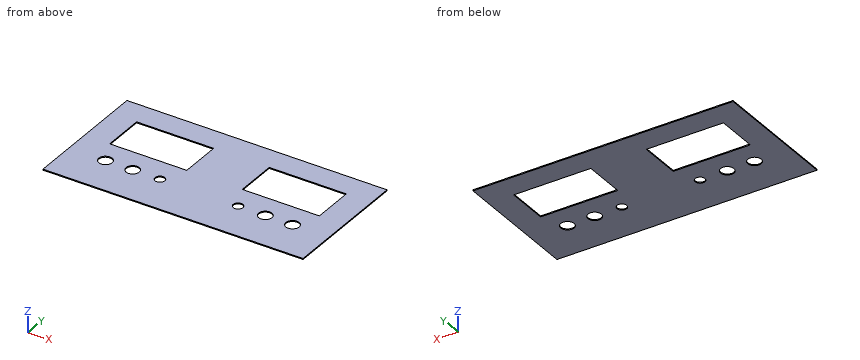
from build123d import *

# Parameters (mm, degrees)
SKETCH1_W          = 253
SKETCH1_H          = 126
BASE_FLANGE1_DEPTH = 1
SKETCH2_R          = 6.5
SKETCH2_R_2        = 4.75
SKETCH2_W          = 75
SKETCH2_H          = 40.400000001
SKETCH2_H_2        = 40.4
CUT_EXTRUDE1_DEPTH = 10


# Sheet-metal steps are written as plain solids
with BuildPart() as part:
    # Sketch1 → Base-Flange1 (new body)
    with BuildSketch(Plane.XY):
        Rectangle(SKETCH1_W, SKETCH1_H)
    extrude(amount=-BASE_FLANGE1_DEPTH)

    # Sketch2 → Cut-Extrude1 (cut)
    with BuildSketch(Plane(origin=(0, 0, -1), x_dir=(-1, 0, 0), z_dir=(0, 0, -1))):
        with Locations((-91, -24)):
            Circle(SKETCH2_R)
        with Locations((-64.5, -24)):
            Circle(SKETCH2_R)
        with Locations((64.5, -24)):
            Circle(SKETCH2_R)
        with Locations((91, -24)):
            Circle(SKETCH2_R)
        with Locations((-38, -24)):
            Circle(SKETCH2_R_2)
        with Locations((38, -24)):
            Circle(SKETCH2_R_2)
        with Locations((-64.5, 19.5)):
            Rectangle(SKETCH2_W, SKETCH2_H)
        with Locations((64.5, 19.5)):
            Rectangle(SKETCH2_W, SKETCH2_H_2)
    extrude(amount=-CUT_EXTRUDE1_DEPTH, mode=Mode.SUBTRACT)


solid = part.part
The model under review builds one solid part; all positions refer to its coordinate system, in mm. Round coordinates to 2 decimals unless told otherwise and drop trailing zeros. Loops run counter-clockwise (first coordinate to the right, second up) from the corner with the lowest first, then second, coordinate; pieces in that order, holes last. Notation, with made-up numbers: M 30.25,32.25 L 71.25,32.25 A9 ccw 71.25,42.25 Z; hole C 38,72 d3. An arc over 180 degrees is marked long. Answer as CSV lines item,"result". Start each with the question number.
Item 1: Consider section A-A (x = 77). Write out the cut boundary in (y, z).
Item 2: Wall thickness on line 1 (X direction, y = 21.5, z = -0.05); line 2 (Y direction, x = -91, z = -0.75); line 3 (Y direction, x = -92, z = -0.25): over which ranges is each line inside the solid? List them lowest first. Write a range as [from, to].
Item 3: Consider section B-B (y = -24). Write out the cut boundary in (x, z), then the cut area to 3 significant figures.
Item 4: Insertion check: P1, Ø10.5, axis at x = 91, y = -24, coming from the +Z side. The pin has a flat end and moves straight along its axis. Give the tip position at first contact, or say it passes through.
Item 5: Consider section D-D (z = -0.6). State how many separate pieces and enclosed holes the cut face has, then the cut area to 3 significant figures.
Item 6: Consider section C-C (x = -91). Write out the cut boundary in (y, z), then the cut area to 3 significant figures.
Answer:
1,outline,"M -63,-1 L -0.7,-1 L -0.7,0 L -63,0 Z; M 39.7,-1 L 63,-1 L 63,0 L 39.7,0 Z"
2,line 1,"x = [-126.5, -102], [-27, 27], [102, 126.5]"
2,line 2,"y = [-63, -30.5], [-17.5, -0.7], [39.7, 63]"
2,line 3,"y = [-63, -30.42], [-17.58, -0.7], [39.7, 63]"
3,outline,"M -126.5,-1 L -97.5,-1 L -97.5,0 L -126.5,0 Z; M -84.5,-1 L -71,-1 L -71,0 L -84.5,0 Z; M -58,-1 L -42.75,-1 L -42.75,0 L -58,0 Z; M -33.25,-1 L 33.25,-1 L 33.25,0 L -33.25,0 Z; M 42.75,-1 L 58,-1 L 58,0 L 42.75,0 Z; M 71,-1 L 84.5,-1 L 84.5,0 L 71,0 Z; M 97.5,-1 L 126.5,-1 L 126.5,0 L 97.5,0 Z"
3,area,"182 mm^2"
4,P1,"passes through"
5,separate pieces,"1"
5,enclosed holes,"8"
5,area,"25,100 mm^2"
6,outline,"M -63,-1 L -30.5,-1 L -30.5,0 L -63,0 Z; M -17.5,-1 L -0.7,-1 L -0.7,0 L -17.5,0 Z; M 39.7,-1 L 63,-1 L 63,0 L 39.7,0 Z"
6,area,"72.6 mm^2"
